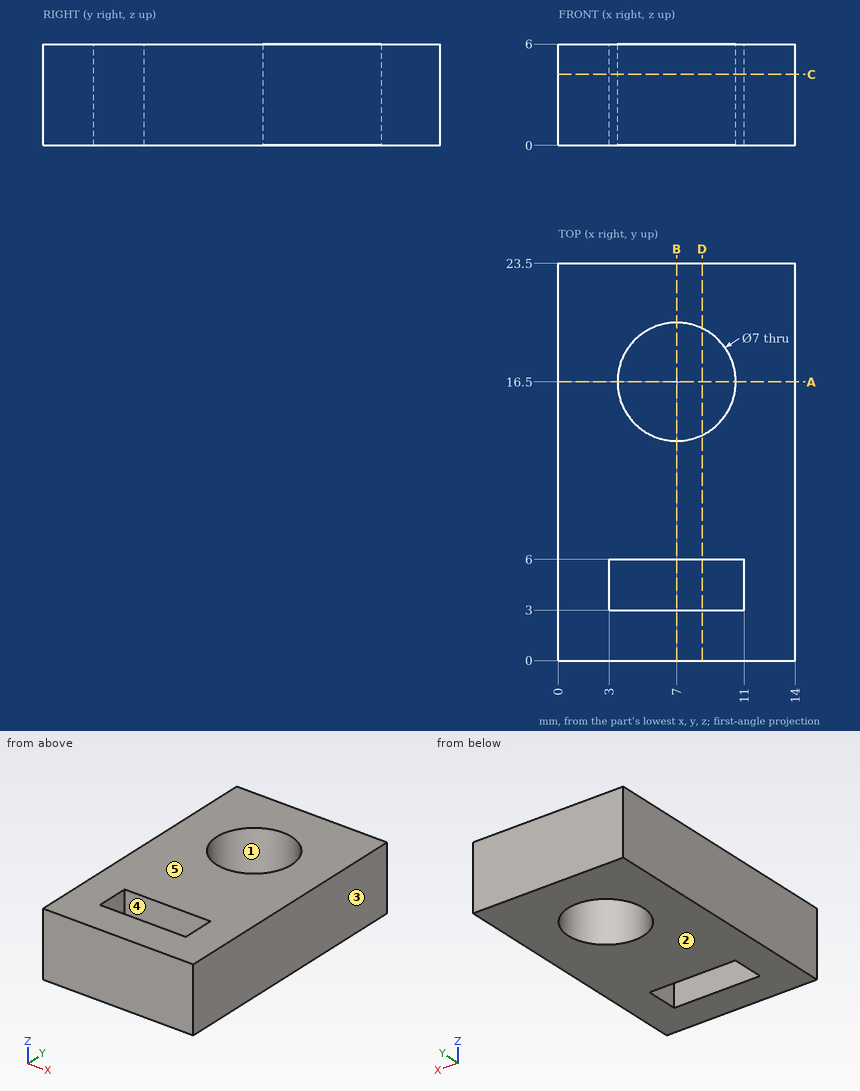
Job drawing, mm, ordinate dimensions from the low corner. One solid piece. A direction names the side the tool comes from. Give positions to 0.01 mm unless a question says otherwise; leave off trailing zeros. Loops run counter-clockwise (first coordinate to the right, second up) from the corner with the lowest first, then second, coordinate; pieces in that order, holes last. Notation, with made-up numbers: M -20,68 L 30,68 A17 cw 30,86 Z; hole C -37.5,76 d1. An arc over 180 degrees is marked long. Return JSON: item names as keys, results as strings.
1) Flat gauge pin, fed straight in: pin 1 Ø6.5 at (x, y) = (7, 16.5) entering from -Z. Where does the tip first touch, or does it go through?
Calculated:
{"pin 1": "passes through"}
2) Saw through at B-B, the plane x = 7. List the corners of the cut face in (y, z), then the cut area to 3 significant figures.
Calculated:
{"outline": "M 0,0 L 3,0 L 3,6 L 0,6 Z; M 6,0 L 13,0 L 13,6 L 6,6 Z; M 20,0 L 23.5,0 L 23.5,6 L 20,6 Z", "area": "81.0 mm2"}
3) 3-axis set-ups, long thin cutter, end or side, ignore diameter. For the marked faces 4 and 5: which of +Z, -Z, +X, -X, +Y, -Y reach the whole face in a straight line?
Calculated:
{"face 4": "+Z, -Z", "face 5": "+Z, +X, -X, +Y, -Y"}
4) Saw through at C-C, the plane z = 4.2. List the corners of the cut face in (x, y), then the cut area to 3 significant figures.
Calculated:
{"outline": "M 0,0 L 14,0 L 14,23.5 L 0,23.5 Z; hole M 3,3 L 11,3 L 11,6 L 3,6 Z; hole C 7,16.5 d7", "area": "267 mm2"}
5) Drill centre lines: line 1 (Y direction, x = 7, z = 2.3); line 2 (X direction, y = 18, z = 2.85); line 3 (Y direction, x = 9.25, z = 2.7). Where is each one in solid material? Low to high.
Calculated:
{"line 1": "y = 0 to 3, 6 to 13, 20 to 23.5", "line 2": "x = 0 to 3.84, 10.16 to 14", "line 3": "y = 0 to 3, 6 to 13.82, 19.18 to 23.5"}
6) Saw through at A-A, the plane y = 16.5. List the corners of the cut face in (x, z), then the cut area to 3 significant figures.
Calculated:
{"outline": "M 0,0 L 3.5,0 L 3.5,6 L 0,6 Z; M 10.5,0 L 14,0 L 14,6 L 10.5,6 Z", "area": "42.0 mm2"}
7) Pull direction X, two halves, no side cores. Call the marked faces 1, 2 and 3: released by +X, released by -X, zero draft, split by the parting line, or undercut.
Calculated:
{"face 1": "undercut", "face 2": "zero draft", "face 3": "released by +X"}
8) Saw through at D-D, the plane x = 8.5. List the corners of the cut face in (y, z), then the cut area to 3 significant figures.
Calculated:
{"outline": "M 0,0 L 3,0 L 3,6 L 0,6 Z; M 6,0 L 13.34,0 L 13.34,6 L 6,6 Z; M 19.66,0 L 23.5,0 L 23.5,6 L 19.66,6 Z", "area": "85.1 mm2"}
